Print and shaded views of the part. All mm, measured from the part's lowest x, y and z. A direction names the side the tool comes from. Round coordinates to 2 decimals unless told otherwise and drop trailing zeros. Write each loop counter-clockwise with the first axis right and the second up, starting at its lowest first coordinate (ties: lowest second). Pieces come first, ordered by that corner, then holes. Notation, with made-up numbers: (31, 19) - (63, 19) arc R17 cw to (63, 28) - close; hole circle Ø7 at (32.5, -0.75). An arc over 180 degrees is marked (long way). One line per item, written item: value.
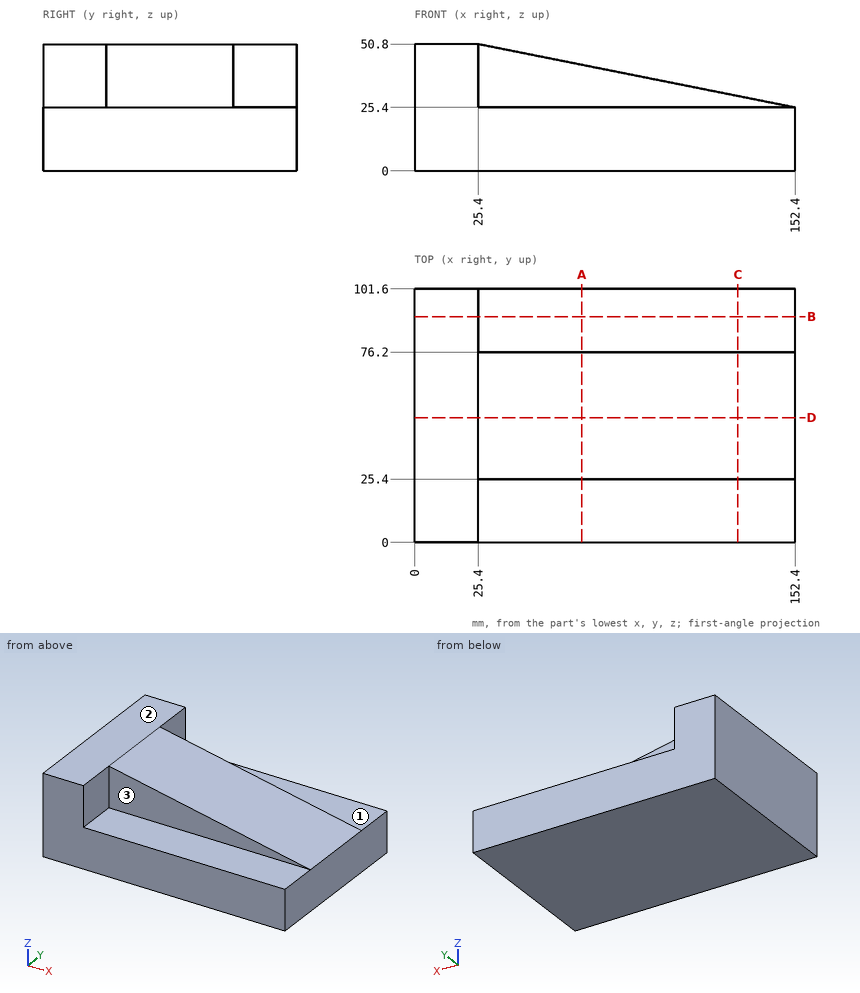
1. Band-saw the part on C-C on x = 129.5. Write the cut outline in (y, z).
Report:
outline: (0, 0) - (101.6, 0) - (101.6, 25.4) - (76.2, 25.4) - (76.2, 29.98) - (25.4, 29.98) - (25.4, 25.4) - (0, 25.4) - close
2. Band-saw the part on A-A on x = 67. Write the cut outline in (y, z), plus the area to 3 significant figures.
Report:
outline: (0, 0) - (101.6, 0) - (101.6, 25.4) - (76.2, 25.4) - (76.2, 42.48) - (25.4, 42.48) - (25.4, 25.4) - (0, 25.4) - close
area: 3,450 mm²
3. Drop flat-ended pins along their axis: pin 1 (6 mm diameter, centred on x = 25.5, y = 69.5, fed in from -Z); pin 2 (1 mm diameter, centred on x = 117, y = 39.5, fed in from +Z); pin 3 (7.5 mm diameter, centred on x = 111, y = 11.5, fed in from +Z); pin 4 (12 mm diameter, centred on x = 69.5, z = 42, fed in from +Y). Give the stop position or say it passes through.
Report:
pin 1: z = 0
pin 2: z = 32.58
pin 3: z = 25.4
pin 4: y = 76.2
4. Tool access for the marked faces 1, 2 and 3: list every direction of +Z, -Z, +X, -X, +Y, -Y with a clear straight run to the whole face (end or side of a thin tool).
Report:
face 1: +Z, +X, +Y
face 2: +Z, +X, -X, +Y, -Y
face 3: +Z, +X, -Y
5. Band-saw the part on D-D on y = 50. Write the cut outline in (x, z), plus the area to 3 significant figures.
Report:
outline: (0, 0) - (152.4, 0) - (152.4, 25.4) - (25.4, 50.8) - (0, 50.8) - close
area: 6,130 mm²
6. Band-saw the part on B-B on y = 90.5. Write the cut outline in (x, z), plus the area to 3 significant figures.
Report:
outline: (0, 0) - (152.4, 0) - (152.4, 25.4) - (25.4, 25.4) - (25.4, 50.8) - (0, 50.8) - close
area: 4,520 mm²
7. Wall check: probe 1 along X at (y, z) = (79.5, 31); probe 2 along Y at (x, z) = (37, 46). Give the ranges that are in metal, low to high. Write a range as [from, to].
Report:
probe 1: [0, 25.4]
probe 2: [25.4, 76.2]
